Part model, mm, in its own coordinate system. Face numbers are marked on the shaded views. A direction names the side the tool comes from. Give positions to 0.01 mm unless a question says otherwise; leave off trailing zeros. Write each loop counter-clockwise with the first axis right and the second up, starting at its lowest first coordinate (ties: lowest second). Pieces come first, ordered by that corner, then holes. Notation, with made-up numbers: M 73.5,86.5 L 114.5,86.5 A24 ccw 114.5,101.5 Z; hole C 82.5,-39.75 d5. An arc over 180 degrees is marked long. Answer as CSV lines item,"result". Start each with the question number.
Item 1: Band-saw the part on A-A, the plane x = 0. List the corners of the cut face in (y, z), then the cut area to 4 significant figures.
Item 2: Two-plate mould, pull along Y, no slides. Class the marked faces 3, 4 and 5: +Y half, -Y half, draft (parallel to the pull), parting line (faces both ways), or undercut.
Item 3: Pin check, flat tip, straight feed: pin 1 (0.8 mm diameter, centred on y = 6, z = 0, fed in from -X). Stop position of the tip, or through.
Item 4: Band-saw the part on B-B, the plane z = 0.35. Count the separate pieces of the cut face and the enclosed holes in it, then the cut area to 3 significant figures.
Item 5: Band-saw the part on C-C, the plane y = 9.5. List the corners of the cut face in (x, z).
Item 6: Wall check: L1, parallel to Y at x = 0, z = 0.85; L2, parallel to X at y = 2, z = 0.5; L3, parallel to X at y = -3, z = -0.1. Give the ranges that are in metal, low to high. Write a range as from..to.
Item 7: 3-axis set-ups, long thin cutter, end or side, ignore diameter. For the marked faces 1 and 2: which of +Z, -Z, +X, -X, +Y, -Y reach the whole face in a straight line?
Item 8: Band-saw the part on D-D, the plane x = -9.75. List the corners of the cut face in (y, z).
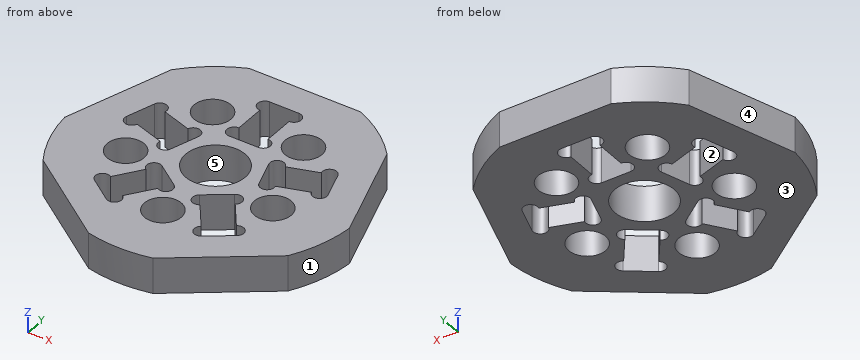
from build123d import *

# Parameters (mm, degrees)
SKETCH_1_R               = 12
EXTRUDE_1_DEPTH          = 1.5
SKETCH_2_R               = 1.55
SKETCH_2_W               = 2.45
SKETCH_2_H               = 5
CUT_EXTRUDE_1_DEPTH      = 4
PATTERN_CIRCULAR_1_COUNT = 5
SKETCH_3_R               = 0.6
CUT_EXTRUDE_2_DEPTH      = 4
PATTERN_CIRCULAR_2_COUNT = 5
SKETCH_4_R               = 2.5
CUT_EXTRUDE_3_DEPTH      = 4
CUT_EXTRUDE_4_DEPTH      = 4
PATTERN_CIRCULAR_3_COUNT = 5


with BuildPart() as part:
    # 草图1 → 凸台-拉伸1 (new body, symmetric)
    with BuildSketch(Plane.XY):
        Circle(SKETCH_1_R)
    extrude(amount=EXTRUDE_1_DEPTH, both=True)

    # 草图2 → 切除-拉伸1 (cut, through all)
    with BuildSketch(Plane.XY.offset(1.5)):
        with Locations((0, -6.5)):
            Circle(SKETCH_2_R)
        with Locations((0, 6)):
            Rectangle(SKETCH_2_W, SKETCH_2_H)
    cut_extrude_1 = extrude(amount=-CUT_EXTRUDE_1_DEPTH, mode=Mode.SUBTRACT)

    # 阵列(圆周)1: 切除-拉伸1 ×5 about axis
    pattern_circular_1_axis = Axis((0, 0, 0), (0, 0, 1))
    for i in range(1, PATTERN_CIRCULAR_1_COUNT):
        add(cut_extrude_1.rotate(pattern_circular_1_axis, i * 360 / PATTERN_CIRCULAR_1_COUNT), mode=Mode.SUBTRACT)

    # 草图3 → 切除-拉伸2 (cut, through all)
    with BuildSketch(Plane.XY.offset(1.5)):
        with Locations((1.225, 7.9)):
            Circle(SKETCH_3_R)
        with Locations((-1.225, 7.9)):
            Circle(SKETCH_3_R)
        with Locations((-1.225, 4.1)):
            Circle(SKETCH_3_R)
        with Locations((1.225, 4.1)):
            Circle(SKETCH_3_R)
    cut_extrude_2 = extrude(amount=-CUT_EXTRUDE_2_DEPTH, mode=Mode.SUBTRACT)

    # 阵列(圆周)2: 切除-拉伸2 ×5 about axis
    pattern_circular_2_axis = Axis((0, 0, 0), (0, 0, 1))
    for i in range(1, PATTERN_CIRCULAR_2_COUNT):
        add(cut_extrude_2.rotate(pattern_circular_2_axis, i * 360 / PATTERN_CIRCULAR_2_COUNT), mode=Mode.SUBTRACT)

    # 草图4 → 切除-拉伸3 (cut, through all)
    with BuildSketch(Plane.XY.offset(1.5)):
        Circle(SKETCH_4_R)
    extrude(amount=-CUT_EXTRUDE_3_DEPTH, mode=Mode.SUBTRACT)

    # 草图5 → 切除-拉伸4 (cut, through all)
    with BuildSketch(Plane.XY.offset(1.5)):
        with BuildLine():
            Line((-4.679476466, 11.05), (4.679476466, 11.05))
            ThreePointArc((4.679476466, 11.05), (0, 12), (-4.679476466, 11.05))
        make_face()
    cut_extrude_4 = extrude(amount=-CUT_EXTRUDE_4_DEPTH, mode=Mode.SUBTRACT)

    # 阵列(圆周)3: 切除-拉伸4 ×5 about axis
    pattern_circular_3_axis = Axis((0, 0, 0), (0, 0, 1))
    for i in range(1, PATTERN_CIRCULAR_3_COUNT):
        add(cut_extrude_4.rotate(pattern_circular_3_axis, i * 360 / PATTERN_CIRCULAR_3_COUNT), mode=Mode.SUBTRACT)


solid = part.part
Output:
1,outline,"M -12,-1.5 L -8.05,-1.5 L -8.05,1.5 L -12,1.5 Z; M -4.95,-1.5 L -2.5,-1.5 L -2.5,1.5 L -4.95,1.5 Z; M 2.5,-1.5 L 3.5,-1.5 L 3.5,1.5 L 2.5,1.5 Z; M 8.5,-1.5 L 11.05,-1.5 L 11.05,1.5 L 8.5,1.5 Z"
1,area,"29.85 mm²"
2,face 3,"draft"
2,face 4,"+Y half"
2,face 5,"undercut"
3,pin 1,"x = -9.8"
4,separate pieces,"1"
4,enclosed holes,"11"
4,area,"293 mm²"
5,outline,"M -7.33,-1.5 L 7.33,-1.5 L 7.33,1.5 L -7.33,1.5 Z"
6,L1,"-12..-8.05, -4.95..-2.5, 2.5..3.5, 8.5..11.05"
6,L2,"-10.97..-8.29, -3.03..-1.5, 1.5..3.03, 8.29..10.97"
6,L3,"-11.62..-7.37, -4.99..-3.85, -1.83..1.83, 3.85..4.99, 7.37..11.62"
7,face 1,"+Z, -Z, +X, -Y"
7,face 2,"+Z, -Z"
8,outline,"M -6.57,-1.5 L 5.75,-1.5 L 5.75,1.5 L -6.57,1.5 Z"
